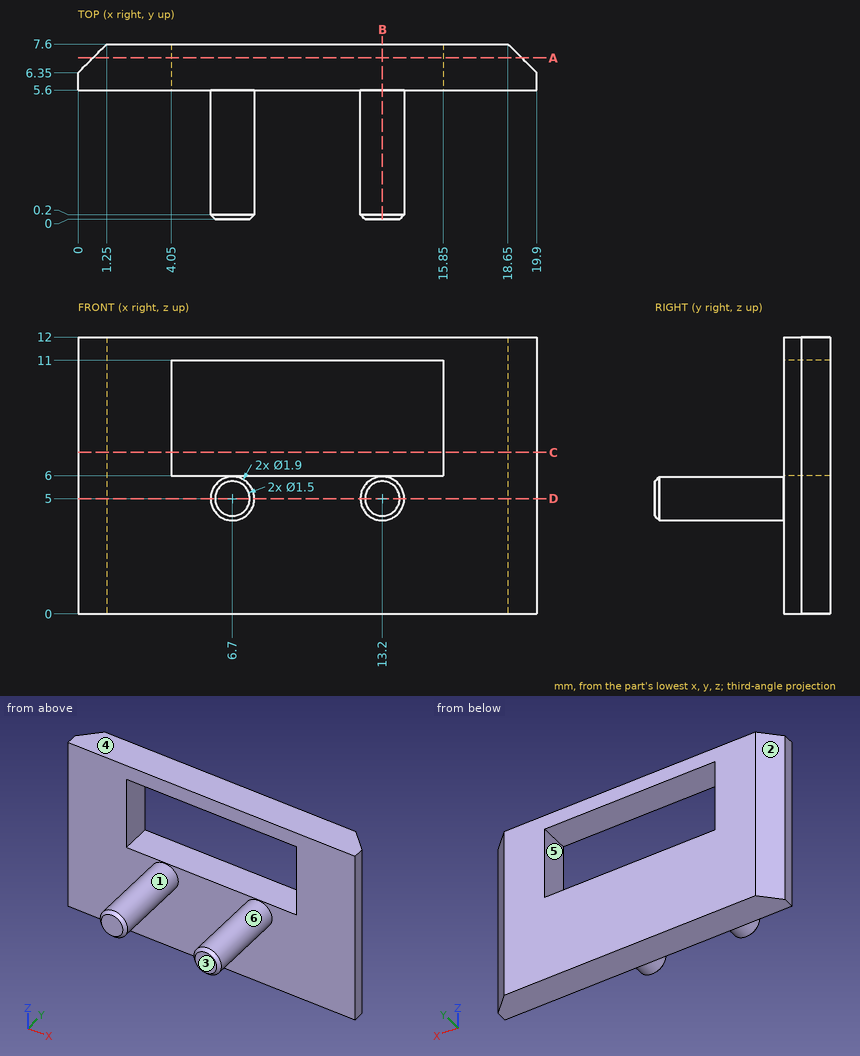
Drawing for the job (mm, zero at the part's lowest x, y, z). A direction names the side the tool comes from. Give positions to 0.01 mm unless a question says otherwise; leave off trailing zeros. Loops run counter-clockwise (first coordinate to the right, second up) from the corner with the lowest first, then second, coordinate; pieces in that order, holes last.
(1) Drill centre lines: line 1 along Z through (x, y) = (14, 6.75); line 2 along X through (y, z) = (6.25, 10); line 3 along Y through (x, z) = (13, 4). Where is each one in solid material? Low to high.
Return value:
line 1: z = 0 to 6, 11 to 12
line 2: x = 0 to 4.05, 15.85 to 19.9
line 3: y = 5.6 to 7.6
(2) Band-saw the part on B-B (x = 13.2). Write the cut outline in (y, z), and give its area (3 significant figures).
Return value:
outline: (0, 4.25) - (0.2, 4.05) - (5.6, 4.05) - (5.6, 0) - (7.6, 0) - (7.6, 6) - (5.6, 6) - (5.6, 5.95) - (0.2, 5.95) - (0, 5.75) - close; (5.6, 11) - (7.6, 11) - (7.6, 12) - (5.6, 12) - close
area: 24.6 mm2
(3) Pin check, flat tips, straight feed: pin 1 (1 mm diameter, centred on y = 2.5, z = 6, fed in from +X); pin 2 (1 mm diameter, centred on x = 12.5, y = 6.5, fed in from -Z); pin 3 (4 mm diameter, centred on x = 4, y = 2.5, fed in from +Z); pin 4 (1 mm diameter, centred on x = 12.5, y = 1, fed in from -Z). Stop position of each tip, or through.
Return value:
pin 1: stops at x = 14.01
pin 2: stops at z = 0
pin 3: stops at z = 5.64
pin 4: stops at z = 4.07
(4) Band-saw the part on C-C (z = 7). Write the cut outline in (x, y), and give its area (3 significant figures).
Return value:
outline: (0, 5.6) - (4.05, 5.6) - (4.05, 7.6) - (1.25, 7.6) - (0, 6.35) - close; (15.85, 5.6) - (19.9, 5.6) - (19.9, 6.35) - (18.65, 7.6) - (15.85, 7.6) - close
area: 14.6 mm2
(5) Pull direction X, two halves, no side cores. Call the marked faces 1, 2 and 3: pulls with the +X half, pulls with the -X half, needs draft (parallel to the pull), parting line crosses it, or undercut.
Return value:
face 1: undercut
face 2: pulls with the -X half
face 3: needs draft
(6) 3-axis set-ups, long thin cutter, end or side, ignore diameter. For the marked faces 4, 5 and 6: which of +Z, -Z, +X, -X, +Y, -Y reach the whole face in a straight line?
Return value:
face 4: +Z, +X, -X, +Y, -Y
face 5: +Y, -Y
face 6: -Y
(7) Band-saw the part on D-D (z = 5). Write the cut outline in (x, y), and give its area (3 significant figures).
Return value:
outline: (0, 5.6) - (5.75, 5.6) - (5.75, 0.2) - (5.95, 0) - (7.45, 0) - (7.65, 0.2) - (7.65, 5.6) - (12.25, 5.6) - (12.25, 0.2) - (12.45, 0) - (13.95, 0) - (14.15, 0.2) - (14.15, 5.6) - (19.9, 5.6) - (19.9, 6.35) - (18.65, 7.6) - (1.25, 7.6) - (0, 6.35) - close
area: 59.4 mm2
(8) Band-saw the part on A-A (y = 7). Write the cut outline in (x, z).
Return value:
outline: (0.65, 0) - (19.25, 0) - (19.25, 12) - (0.65, 12) - close; hole (4.05, 6) - (15.85, 6) - (15.85, 11) - (4.05, 11) - close
